Part model, mm, in its own coordinate system. Face numbers are marked on the shaded views. A direction names the side the tool comes from. Round coordinates to 2 decimals unless told otherwise and drop trailing zeros. Order: outer loops, then holes, each group sorted by start corner. A loop starts at its lowest first (then second) coordinate and runs counter-clockwise, first axis right, second up. Notation, with made-up numbers: (28.25, 38) - (57.25, 38) arc R19 ccw to (57.25, 44) - close; hole circle Ø6 at (-12.75, 15). An arc over 180 degrees is marked (long way). Return JSON: item names as keys, results as strings. Group by question number.
Item 1: Probe probe 1 along Y at (x, z) = (-32, 25.5); probe 2 along X at (y, z) = (-13, 41); probe 3 along Z at (x, y) = (-44, -19.5). List the from-to ranges inside material, lowest first.
Item 2: Saw through at C-C on x = -5. List the corners of the cut face in (y, z), and give its area (3 significant figures).
Item 3: Saw through at A-A on y = -23.5. List the corners of the cut face in (x, z).
Item 4: Tool access for the marked faces 4, 5 and 6: list every direction of +Z, -Z, +X, -X, +Y, -Y with a clear straight run to the whole face (end or side of a thin tool).
Item 5: Two-plate mould, pull along X, no slides. Class the marked faces 1, 2 and 3: released by +X, released by -X, zero draft, split by the parting line, or undercut.
Item 6: Drop flat-ended pins along their axis: pin 1 (7.5 mm diameter, centred on y = -17, z = 40, fed in from -X); pin 2 (5 mm diameter, centred on x = -21, z = 11.5, fed in from -Y); pin 3 (7.5 mm diameter, centred on x = -59, y = -17, fed in from +Z); pin 4 (2 mm diameter, centred on x = -36.5, y = -27, fed in from +Z). Give the stop position or say it passes through.
Item 7: Saw through at B-B on z = 42. List the corners of the cut face in (x, y), and give its area (3 significant figures).
Item 8: Saw through at D-D on z = 11. List the corners of the cut face in (x, y).
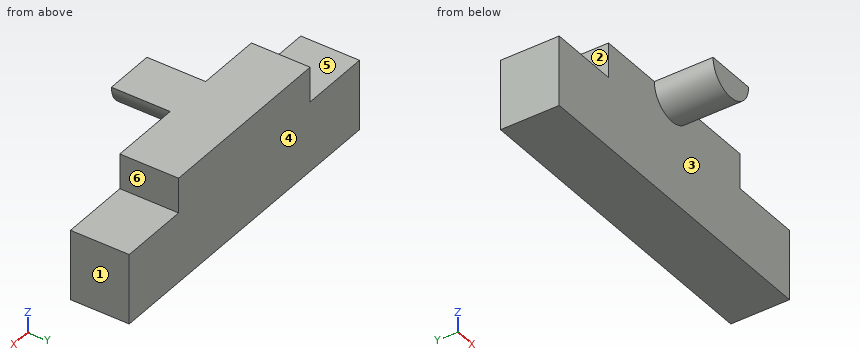
```python
from build123d import *

# Parameters (mm, degrees)
F1_DEPTH = 25
F3_DEPTH = 25


with BuildPart() as f1:
    # F0 (on Front) → F1 (new body)
    with BuildSketch(Plane.XZ):
        Polygon((-68.520491, 30), (-68.520491, 0), (71.479509, 0), (71.479509, 30), (41.479509, 30), (41.479509, 45), (-38.520491, 45), (-38.520491, 30), align=None)
    extrude(amount=F1_DEPTH)

    # F2 (on face) → F3 (join)
    with BuildSketch(Plane.XZ.offset(25)):
        with BuildLine():
            ThreePointArc((-10.685148, 45), (0.05549, 34.113566), (10.893544, 44.903021))
            ThreePointArc((10.893544, 44.903021), (10.893435, 44.951511), (10.893108, 45))
            Line((10.893108, 45), (-10.685148, 45))
        make_face()
    extrude(amount=F3_DEPTH)


solid = f1.part
```
Filled in:
{
 "1": {"probe 1": "y = -25 to 0", "probe 2": "x = -38.52 to 41.48", "probe 3": "z = 0 to 30"},
 "2": {"outline": "(-50, 35.4) - (-25, 35.4) - (-25, 0) - (0, 0) - (0, 45) - (-50, 45) - close", "area": "1,370 mm^2"},
 "3": {"outline": "(-68.52, 0) - (71.48, 0) - (71.48, 30) - (41.48, 30) - (41.48, 45) - (-38.52, 45) - (-38.52, 30) - (-68.52, 30) - close"},
 "4": {"face 4": "+Z, -Z, +X, -X, +Y", "face 5": "+Z, -X, +Y, -Y", "face 6": "+Z, +X, +Y, -Y"},
 "5": {"face 1": "released by +X", "face 2": "released by -X", "face 3": "zero draft"},
 "6": {"pin 1": "stops at x = -38.52", "pin 2": "stops at y = -25", "pin 3": "stops at z = 30", "pin 4": "passes through"},
 "7": {"outline": "(-38.52, -25) - (-10.29, -25) - (-10.29, -50) - (10.5, -50) - (10.5, -25) - (41.48, -25) - (41.48, 0) - (-38.52, 0) - close", "area": "2,520 mm^2"},
 "8": {"outline": "(-68.52, -25) - (71.48, -25) - (71.48, 0) - (-68.52, 0) - close"}
}
